Work out the finished part from the listing and answer in its coordinate system (mm). Face numbers are marked on the shaded views. Coordinates: 2 decimals unless noted, no trailing zeros. Write each loop counter-clockwise with the first axis right and the second up, starting at its lowest first coordinate (ties: lowest second). Pieces come first, ordered by that corner, then holes. Notation, with made-up numbers: (63, 2) - (81, 2) arc R22 cw to (81, 27) - close; hole circle Ø1 at (8.25, 45). An arc over 180 degrees is marked (long way). Use one line per item in the form item = value. Start each with the question number.
Item 1: Given pin 1 (3.5 mm diameter, centred on x = 5, y = 60, fed in from -Z); pin 2 (2 mm diameter, centred on y = 10, z = 6, fed in from +X); pin 3 (2.5 mm diameter, centred on x = 5, y = 39.5, fed in from -Z), each flat-ended and moving along its own axis, determine where each tip first touches the part or whether it passes through.
Item 2: Determine the mould class of the marked faces 1, 2, 3 and 4 for opening direction Y: released by +Y, released by -Y, zero draft, split by the parting line, or undercut.
Item 3: A cutting plane is placed at A-A (z = 5.75). Write down the section's boundary in (x, y).
Item 4: A cutting plane is placed at C-C (y = 92.5). Write down the section's boundary in (x, z), then the cut area to 3 significant figures.
Item 5: A cutting plane is placed at D-D (y = 60). Write down the section's boundary in (x, z).
Item 6: A cutting plane is placed at B-B (x = 5). Write down the section's boundary in (y, z), then the cut area to 3 significant figures.
Item 7: Consider probe 1 along Y at (x, z) = (7.25, 5.75); probe 2 along X at (y, z) = (39.5, 7); probe 3 along Y at (x, z) = (5, 6.5). Determine where each line is inside the solid, lowest interval first.
Autodesk Inventor part; units mm, degrees
ref_plane "YZ Plane" through (0, 0, 0) normal (1, 0, 0) x (0, 1, 0)
ref_plane "XZ Plane" through (0, 0, 0) normal (0, 1, 0) x (-1, 0, 0)
ref_plane "XY Plane" through (0, 0, 0) normal (0, 0, 1) x (1, 0, 0)
sketch "Sketch1" plane through (0, 0, 0) normal (0, 0, 1) x (1, 0, 0)
  line L0 (0, 0) -> (10, 0)
  line L1 (10, 0) -> (10, 100)
  line L2 (10, 100) -> (0, 100)
  line L3 (0, 100) -> (0, 0)
  dimension "d0" = 10
  dimension "d1" = 100
extrude "Extrusion1" add sketch "Sketch1" along normal blind 11.5
sketch "Sketch2" plane through (0, 0, 11.5) normal (0, 0, 1) x (1, 0, 0)
  line L0 (10, 100) -> (0, 100)
  line L1 (0, 0) -> (10, 0)
  point P0 (5, 39.5)
  point P1 (5, 60)
  point P2 (5, 100)
  dimension "d4" = 20.5
  dimension "d5" = 40
  dimension "d14" = 39.5
  dimension "d24" = 100
hole "Hole1" at (5, 39.5, 11.5) at (5, 60, 11.5) direction (0, 0, -1) diameter 3.242 end through all
sketch "Sketch3" plane through (10, 0, 0) normal (1, 0, 0) x (0, 0, -1)
  line L0 (0, 100) -> (-11.5, 100)
  line L1 (0, 0) -> (-11.5, 0)
  point P0 (-5.75, 92.5)
  point P1 (-5.75, 7.5)
  point P2 (-5.75, 100)
  dimension "d15" = 7.5
  dimension "d16" = 7.5
hole "Hole2" at (10, 92.5, 5.75) at (10, 7.5, 5.75) direction (-1, 0, 0) diameter 4.5 end through all countersink diameter 9.4 countersink angle 90
properties part number "Pancake_Flexi Pipe Mount" material "Aluminum 6061"
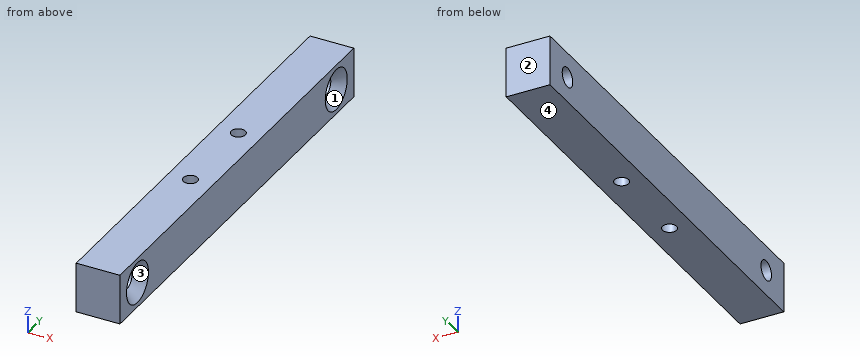
Answer:
q1.pin_1 = 0
q1.pin_2 = 8.81
q1.pin_3 = through
q2.face_1 = undercut
q2.face_2 = released by +Y
q2.face_3 = undercut
q2.face_4 = zero draft
q3.outline = (0, 0) - (10, 0) - (10, 2.8) - (7.55, 5.25) - (0, 5.25) - close; (0, 9.75) - (7.55, 9.75) - (10, 12.2) - (10, 87.8) - (7.55, 90.25) - (0, 90.25) - close; (0, 94.75) - (7.55, 94.75) - (10, 97.2) - (10, 100) - (0, 100) - close; hole circle Ø3.24 at (5, 39.5); hole circle Ø3.24 at (5, 60)
q4.outline = (0, 0) - (10, 0) - (10, 1.05) - (7.55, 3.5) - (0, 3.5) - close; (0, 8) - (7.55, 8) - (10, 10.45) - (10, 11.5) - (0, 11.5) - close
q4.area = 64.0 mm²
q5.outline = (0, 0) - (3.38, 0) - (3.38, 11.5) - (0, 11.5) - close; (6.62, 0) - (10, 0) - (10, 11.5) - (6.62, 11.5) - close
q6.outline = (0, 0) - (37.88, 0) - (37.88, 11.5) - (0, 11.5) - close; (41.12, 0) - (58.38, 0) - (58.38, 11.5) - (41.12, 11.5) - close; (61.62, 0) - (100, 0) - (100, 11.5) - (61.62, 11.5) - close; hole circle Ø4.5 at (7.5, 5.75); hole circle Ø4.5 at (92.5, 5.75)
q6.area = 1,040 mm²
q7.probe_1 = 0 to 5.25, 9.75 to 90.25, 94.75 to 100
q7.probe_2 = 0 to 3.38, 6.62 to 10
q7.probe_3 = 0 to 5.38, 9.62 to 37.88, 41.12 to 58.38, 61.62 to 90.38, 94.62 to 100
